Could you check a few things on this model? Use its own coordinates, in mm. A direction names the side the tool comes from. Coordinates: 2 decimals unless noted, no trailing zeros. One line per question, with ' | ' between items. Start each with the question number.
(1) Which directions (+Z, -Z, +X, -X, +Y, -Y) give clear straight access to the entire face, cutting with the end or side of a thin tool? Please do faces 1 (the face through (0, 6, 4)), 2 (the face through (47, -2, -3)).
(2) I'm going to push flat-ended pins straight in: pin 1 Ø4 at (y, z) = (23.5, 54) entering from -X; pin 2 Ø3.5 at (x, z) = (-3, 57.5) entering from +Y; pin 3 Ø3 at (x, z) = (36, -132.5) entering from +Y. Where does each tip first touch, or does it pass through?
(3) If I drill on line 1 along X through (y, z) = (-25, 135.5); line 2 along Y through (x, z) = (22.5, -153.5); line 3 along X through (y, z) = (42.5, -242.5), over which ranges is the centre line in solid material (lowest first)?
Autodesk Inventor part; units mm, degrees
ref_plane "Work Plane1" through (47, 0, 0) normal (1, 0, 0) x (0, 0, -1)
ref_plane "YZ Plane" through (0, 0, 0) normal (1, 0, 0) x (0, 1, 0)
ref_plane "XZ Plane" through (0, 0, 0) normal (0, 1, 0) x (-1, 0, 0)
sketch "Sketch1" plane through (0, 0, 0) normal (1, 0, 0) x (0, 1, 0)
  line L0 (-161.65, 269.7) -> (161.65, 269.7)
  line L1 (161.65, 269.7) -> (161.65, -269.7)
  line L2 (161.65, -269.7) -> (-161.65, -269.7)
  line L3 (-161.65, -269.7) -> (-161.65, 269.7)
  line L4 (-161.65, 269.7) -> (161.65, -269.7) construction
  line L5 (161.65, 269.7) -> (-161.65, -269.7) construction
  point P0 (0, 0)
  dimension "d0" = 323.3
  dimension "d1" = 539.4
extrude "Extrusion1" add sketch "Sketch1" along normal blind 10
ref_plane "Work Plane1" through (47, 0, 0) normal (1, 0, 0) x (0, 0, -1)
sketch "Sketch2" plane through (47, 0, 0) normal (1, 0, 0) x (0, 0, -1)
  line L0 (-142.5, 69.9526) -> (142.5, 69.9526)
  line L1 (142.5, 69.9526) -> (142.5, -73.0474)
  line L2 (142.5, -73.0474) -> (-142.5, -73.0474)
  line L3 (-142.5, -73.0474) -> (-142.5, 69.9526)
  line L4 (-142.5, 69.9526) -> (142.5, -73.0474) construction
  line L5 (142.5, 69.9526) -> (-142.5, -73.0474) construction
  point P0 (0, 0)
  point P1 (0, -1.5474)
  dimension "d5" = 285
  dimension "d6" = 143
sketch "Sketch3" plane through (10, 0, 0) normal (1, 0, 0) x (0, 0, -1)
  line L0 (269.7, -161.65) -> (269.7, 161.65)
  line L1 (269.7, 161.65) -> (-269.7, 161.65)
  line L2 (-269.7, 161.65) -> (-269.7, -161.65)
  line L3 (-269.7, -161.65) -> (269.7, -161.65)
  point P0 (0, 0)
loft "Loft1" add profiles "Sketch2" section 1 edges at (10, 0, -269.7) (10, 161.65, 0) (10, 0, 269.7) (10, -161.65, 0)
sketch "Sketch4" plane through (0, 0, 0) normal (-1, 0, 0) x (0, 0, 1)
  line L0 (-269.7, -161.65) -> (-269.7, 161.65)
  line L1 (269.7, -161.65) -> (-269.7, -161.65)
  line L2 (269.7, 161.65) -> (269.7, -161.65)
  line L3 (-269.7, 161.65) -> (269.7, 161.65)
  line L4 (-269.7, -161.65) -> (-269.7, 161.65)
  line L5 (-269.7, -145.2634) -> (269.7, -145.2634)
  point P0 (0, 0)
extrude "Extrusion2" add sketch "Sketch4" along normal blind 7 contours L0 L5 L2 L1
properties part number "PANTALLA" material "Steel, Mild, Welded"
Checks:
1) face 1: +Z, -Z, -X, +Y | face 2: +Z, -Z, +X, +Y, -Y
2) pin 1: stops at x = 0 | pin 2: stops at y = -145.26 | pin 3: stops at y = 100.93
3) line 1: x = 0 to 47 | line 2: y = -131.72 to 130.67 | line 3: x = 0 to 17.91
